Read the model definition and answer for the solid it produces. Units are mm, in the model's axes. A direction names the side the tool comes from. Coordinates: 2 decimals unless noted, no trailing zeros. Write each loop counter-clockwise with the first axis right and the second up, starting at its lowest first coordinate (ties: lowest second). Pieces come first, ordered by that corner, then holes.
Item 1: Section A-A (y = -2.25) is taken. Give the vertices of the cut face in (x, z), then the cut area to 3 significant figures.
Item 2: Section C-C (x = 12.75) is taken. Give the vertices of the cut face in (y, z), then the cut area to 3 significant figures.
Item 3: A tool of negligible diameter and unlimited length cuts with its end or side. For faces 1 (the face through (10.25, -9, 12)), 2 (the face through (0, -4, 15)), 3 (the face through (0, -5, -6)), from which of +Z, -Z, +X, -X, +Y, -Y can it reach the whole face along a straight path? Write none if from no direction.
Item 4: Straight lines are drawn through the part: probe 1 along X at (y, z) = (-1.5, -10); probe 2 along X at (y, z) = (-9.5, 11.5); probe 3 along Y at (x, z) = (5, -0.75). For each, find the intervals that lie inside material, in ascending order.
Item 5: Determine the mould class of faces 4 (the face through (-10.25, -9, 11)), 5 (the face through (15, -4, 3)), 6 (the face through (0, -9, 3)) for opening direction X: released by +X, released by -X, zero draft, split by the parting line, or undercut.
Item 6: Section D-D (x = 0.5) is taken. Give the vertices of the cut face in (y, z), then the cut area to 3 significant figures.
Item 7: Section B-B (z = -3) is taken. Give the vertices of the cut face in (x, y), then the cut area to 3 significant figures.
Item 8: Each of these flat-tipped pins is pushed along its axis until it touches: P1, Ø1.5, axis at x = 8.5, z = -4.5, coming from the +Y side; P2, Ø3.5, axis at x = 0, z = -10, coming from the -Y side; P3, Ø1, axis at x = 5, y = -8.5, coming from the +Z side; P4, Ø2.5, axis at x = 7, y = -7.5, coming from the -Z side. Where does it stop, or does it pass through?
from build123d import *

# Parameters (mm, degrees)
F0_W     = 30
F0_H     = 30
F1_DEPTH = 5
F3_W     = 20.5
F3_H     = 5
F4_DEPTH = 8
F6_DEPTH = 25


with BuildPart() as f1:
    # F0 (on Front) → F1 (new body)
    with BuildSketch(Plane.XZ):
        Rectangle(F0_W, F0_H)
    extrude(amount=F1_DEPTH)

    # F3 (on face) → F4 (join)
    with BuildSketch(Plane.XZ.offset(5)):
        Polygon((-10.25, 8), (-10.25, 15), (-15, 15), (-15, 3), (-10.25, 3), align=None)
        with Locations((0, 5.5)):
            Rectangle(F3_W, F3_H)
        Polygon((15, 15), (10.25, 15), (10.25, 8), (10.25, 3), (15, 3), align=None)
    extrude(amount=F4_DEPTH)

    # F5 (on face) → F6 (cut)
    with BuildSketch(Plane.XZ.offset(5)):
        with BuildLine():
            Line((0, -2), (0, -0.45))
            ThreePointArc((0, -0.45), (-1.55, -2), (0, -3.55))
            Line((0, -3.55), (0, -2))
        make_face()
        with BuildLine():
            ThreePointArc((1.55, -2), (1.0960155108, -0.9039844892), (0, -0.45))
            Line((0, -0.45), (0, -2))
            Line((0, -2), (0, -3.55))
            ThreePointArc((0, -3.55), (1.0960155108, -3.0960155108), (1.55, -2))
        make_face()
        with BuildLine():
            ThreePointArc((1.55, -10), (1.0960155108, -8.9039844892), (0, -8.45))
            ThreePointArc((0, -8.45), (-1.0960155108, -11.0960155108), (1.55, -10))
        make_face()
    extrude(amount=-F6_DEPTH, mode=Mode.SUBTRACT)


solid = f1.part
Established:
1. outline: (-15, -15) - (15, -15) - (15, 15) - (-15, 15) - close; hole circle Ø3.1 at (0, -10); hole circle Ø3.1 at (0, -2)
1. area: 885 mm2
2. outline: (-13, 3) - (-5, 3) - (-5, -15) - (0, -15) - (0, 15) - (-13, 15) - close
2. area: 246 mm2
3. face 1: +Z, -Y
3. face 2: +Z, +X, -X, +Y, -Y
3. face 3: -Z, +X, -X, -Y
4. probe 1: x = -15 to -1.55, 1.55 to 15
4. probe 2: x = -15 to -10.25, 10.25 to 15
4. probe 3: y = -5 to 0
5. face 4: undercut
5. face 5: released by +X
5. face 6: zero draft
6. outline: (-13, 3) - (-5, 3) - (-5, -0.53) - (0, -0.53) - (0, 15) - (-5, 15) - (-5, 8) - (-13, 8) - close; (-5, -15) - (0, -15) - (0, -11.47) - (-5, -11.47) - close; (-5, -8.53) - (0, -8.53) - (0, -3.47) - (-5, -3.47) - close
6. area: 161 mm2
7. outline: (-15, -5) - (-1.18, -5) - (-1.18, 0) - (-15, 0) - close; (1.18, -5) - (15, -5) - (15, 0) - (1.18, 0) - close
7. area: 138 mm2
8. P1: stops at y = 0
8. P2: stops at y = -5
8. P3: stops at z = 8
8. P4: stops at z = 3
